from build123d import *

# Parameters (mm, degrees)
F0_R     = 53.6605194211
F1_DEPTH = 25.4
F3_DEPTH = 32.2364754975


with BuildPart() as f1:
    # F0 (on Front) → F1 (new body)
    with BuildSketch(Plane.XZ):
        with Locations((53.6605194211, 0)):
            Circle(F0_R)
    extrude(amount=F1_DEPTH)

    # F2 (on face) → F3 (join)
    with BuildSketch(Plane(origin=(0, 0, 0), x_dir=(-1, 0, 0), z_dir=(0, 1, 0))):
        with BuildLine():
            Line((-49.6755093336, 24.3517733055), (-49.6755093336, 0))
            Line((-49.6755093336, 0), (0, 0))
            ThreePointArc((0, 0), (-14.3331176779, 36.5076268289), (-49.6755093336, 53.512344736))
            Line((-49.6755093336, 53.512344736), (-49.6755093336, 24.3517733055))
        make_face()
        Polygon((-101.477278841, -6.7454725504), (-49.6755093336, -6.7454725504), (-49.6755093336, 0), (-49.6755093336, 24.3517733055), (-101.477278841, 24.3517733055), align=None)
        with BuildLine():
            Line((-46.5558620227, -33.2158250568), (-49.6755093336, -33.2158250568))
            Line((-49.6755093336, -33.2158250568), (-95.8050363876, -33.2158250568))
            ThreePointArc((-95.8050363876, -33.2158250568), (-80.2329364873, -46.6192878088), (-60.7651768195, -53.1881113388))
            Line((-60.7651768195, -53.1881113388), (-46.5558620227, -53.1881113388))
            Line((-46.5558620227, -53.1881113388), (-46.5558620227, -33.2158250568))
        make_face()
    extrude(amount=F3_DEPTH)


solid = f1.part
Geometry check sheet. Reference: the model listing, model coordinates, mm. A direction names the side the tool comes from. Round coordinates to 2 decimals unless told otherwise and drop trailing zeros. Loops run counter-clockwise (first coordinate to the right, second up) from the corner with the lowest first, then second, coordinate; pieces in that order, holes last.
Item 1: Mould release check, pull along Z, two halves, no side actions. Record for faces 6 (the flat face through (75, 16, 24.352)), 7 (the flat face through (54, 16, -53.188)), 8 (the flat face through (51, 32.236, 17)), 9 (the flat face through (49.676, 16, -3)): pulls with the +Z half, pulls with the -Z half, needs draft (parallel to the pull), parting line crosses it, or undercut.
Item 2: Cross-section at D-D on y = -21. Record the boundary of the cut face in (x, z).
Item 3: Gauge pin test, flat ends, axial feed: pin 1 (1 mm diameter, centred on x = 34, y = -7, fed in from +Z); pin 2 (1 mm diameter, centred on y = -13.5, z = 41.5, fed in from +X); pin 3 (9.5 mm diameter, centred on x = 71.5, y = 17, fed in from +Z). Record the tip position at first contact, or that the pin passes through.
Item 4: Cross-section at C-C on z = 21.5. Record the boundary of the cut face in (x, y).
Item 5: Cross-section at B-B on x = 27.5. Record the boundary of the cut face in (y, z), then the cut area to 3 significant figures.
Item 6: Thickness scan on line 1 (Y direction, x = 76, z = 39.5); line 2 (Z direction, x = 71, y = 3); line 3 (Z direction, x = 47, y = 25). Record the ranges inside material, lowest first.
Item 7: Access from +Z, -Z, +X, -X, +Y, -Y to the whole of each face (thin tool, end or side, straight path). Record for faces 1 (the flat face through (46.556, 16, -43)), 2 (the flat face through (101.477, 16, 9)), 3 (the flat face through (76, 16, -6.745)), 4 (the flat face through (66, 32.236, -41)), 5 (the flat face through (49.676, 16, 39)).
Item 8: Cross-section at A-A on y = 14. Record the boundary of the cut face in (x, z).
Answer sheet:
1. face 6: pulls with the +Z half
1. face 7: pulls with the -Z half
1. face 8: needs draft
1. face 9: undercut
2. outline: circle Ø107.32 at (53.66, 0)
3. pin 1: stops at z = 50.12
3. pin 2: stops at x = 88.28
3. pin 3: stops at z = 24.35
4. outline: (4.5, -25.4) - (102.83, -25.4) - (102.83, 0) - (101.48, 0) - (101.48, 32.24) - (4.5, 32.24) - close
5. outline: (-25.4, -46.85) - (0, -46.85) - (0, 0) - (32.24, 0) - (32.24, 46.85) - (-25.4, 46.85) - close
5. area: 3,890 mm2
6. line 1: y = -25.4 to 0
6. line 2: z = -50.78 to -33.22, -6.75 to 24.35
6. line 3: z = -53.19 to -33.22, 0 to 53.25
7. face 1: -Z, -X, +Y
7. face 2: +Z, -Z, +X, +Y
7. face 3: +X, -X, +Y
7. face 4: +Z, -Z, +X, -X, +Y
7. face 5: +Z, +X, +Y
8. outline: (0, 0) - (49.68, 0) - (49.68, -6.75) - (101.48, -6.75) - (101.48, 24.35) - (49.68, 24.35) - (49.68, 53.51) arc R53.66 ccw to start; (46.56, -53.19) - (60.77, -53.19) arc R53.66 ccw to (95.81, -33.22) - (46.56, -33.22) - close
